Source: CAD feature listing. Evaluate the final solid. Frame: model axes, mm. A direction names the side the tool comes from. Round coordinates to 2 decimals unless told otherwise and drop trailing zeros. Loops run counter-clockwise (first coordinate to the right, second up) from the corner with the lowest first, then second, coordinate; pieces in that order, holes last. Notation, with made-up numbers: (-16, 49.5) - (6, 49.5) arc R20 cw to (6, 58.5) - close; hole circle Ø8 at (-30.5, 77.5). An arc over 180 degrees is marked (long way). One line per question, with ' | ' between items.
from build123d import *

# Parameters (mm, degrees)
SKIZZE1_W                       = 168
SKIZZE1_H                       = 60
AUFSATZ_LINEAR_AUSTRAGEN1_DEPTH = 10
SKIZZE2_R                       = 14
SCHNITT_LINEAR_AUSTRAGEN1_DEPTH = 27
SKIZZE3_R                       = 16
SCHNITT_LINEAR_AUSTRAGEN2_DEPTH = 8
SKIZZE4_R                       = 11
SCHNITT_LINEAR_AUSTRAGEN3_DEPTH = 21.6
SKIZZE5_W                       = 168
SKIZZE5_H                       = 10
AUFSATZ_LINEAR_AUSTRAGEN2_DEPTH = 50
SKIZZE6_R                       = 2
SCHNITT_LINEAR_AUSTRAGEN4_DEPTH = 10
SKIZZE7_R                       = 2.5
SCHNITT_LINEAR_AUSTRAGEN5_DEPTH = 10
SKIZZE8_R                       = 1.5
SCHNITT_LINEAR_AUSTRAGEN6_DEPTH = 27
FASE1_SIZE                      = 2
FASE2_SIZE                      = 2
FASE3_SIZE                      = 2
FASE4_SIZE                      = 2


with BuildPart() as part:
    # Skizze1 → Aufsatz-Linear austragen1 (new body)
    with BuildSketch(Plane.XY):
        with Locations((84, 30)):
            Rectangle(SKIZZE1_W, SKIZZE1_H)
    extrude(amount=AUFSATZ_LINEAR_AUSTRAGEN1_DEPTH)

    # Skizze2 → Schnitt-Linear austragen1 (cut)
    with BuildSketch(Plane.XY.offset(10)):
        with Locations((108, 32.5)):
            Circle(SKIZZE2_R)
    extrude(amount=-SCHNITT_LINEAR_AUSTRAGEN1_DEPTH, mode=Mode.SUBTRACT)

    # Skizze3 → Schnitt-Linear austragen2 (cut)
    with BuildSketch(Plane.XY.offset(10)):
        with Locations((108, 32.5)):
            Circle(SKIZZE3_R)
    extrude(amount=-SCHNITT_LINEAR_AUSTRAGEN2_DEPTH, mode=Mode.SUBTRACT)

    # Skizze4 → Schnitt-Linear austragen3 (cut)
    with BuildSketch(Plane(origin=(0, 0, 0), x_dir=(-1, 0, 0), z_dir=(0, 0, -1))):
        with Locations((-66, 32.50089026)):
            Circle(SKIZZE4_R)
    extrude(amount=-SCHNITT_LINEAR_AUSTRAGEN3_DEPTH, mode=Mode.SUBTRACT)

    # Skizze5 → Aufsatz-Linear austragen2 (add)
    with BuildSketch(Plane(origin=(0, 0, 0), x_dir=(-1, 0, 0), z_dir=(0, 0, -1))):
        with Locations((-84, 5)):
            Rectangle(SKIZZE5_W, SKIZZE5_H)
    extrude(amount=AUFSATZ_LINEAR_AUSTRAGEN2_DEPTH)

    # Skizze6 → Schnitt-Linear austragen4 (cut)
    with BuildSketch(Plane(origin=(0, 10, 0), x_dir=(1, 0, 0), z_dir=(0, 1, 0))):
        with Locations((5.5, 13.5)):
            Circle(SKIZZE6_R)
        with Locations((31.5, 13.5)):
            Circle(SKIZZE6_R)
        with Locations((162.5, 13.5)):
            Circle(SKIZZE6_R)
        with Locations((136.5, 13.5)):
            Circle(SKIZZE6_R)
    extrude(amount=-SCHNITT_LINEAR_AUSTRAGEN4_DEPTH, mode=Mode.SUBTRACT)

    # Skizze7 → Schnitt-Linear austragen5 (cut)
    with BuildSketch(Plane(origin=(0, 10, 0), x_dir=(1, 0, 0), z_dir=(0, 1, 0))):
        with Locations((104, 20)):
            Circle(SKIZZE7_R)
        with Locations((64, 20)):
            Circle(SKIZZE7_R)
        with Locations((64, 5)):
            Circle(SKIZZE7_R)
        with Locations((104, 5)):
            Circle(SKIZZE7_R)
    extrude(amount=-SCHNITT_LINEAR_AUSTRAGEN5_DEPTH, mode=Mode.SUBTRACT)

    # Skizze8 → Schnitt-Linear austragen6 (cut)
    with BuildSketch(Plane(origin=(0, 0, 0), x_dir=(-1, 0, 0), z_dir=(0, 0, -1))):
        with Locations((-50.5, 48)):
            Circle(SKIZZE8_R)
        with Locations((-50.5, 17)):
            Circle(SKIZZE8_R)
        with Locations((-81.5, 17)):
            Circle(SKIZZE8_R)
        with Locations((-81.5, 48)):
            Circle(SKIZZE8_R)
    extrude(amount=-SCHNITT_LINEAR_AUSTRAGEN6_DEPTH, mode=Mode.SUBTRACT)

    # Fase1
    fase1_edges = [part.edges().sort_by_distance(p)[0] for p in [
        (61.5, 10, -5),
    ]]
    chamfer(fase1_edges, length=FASE1_SIZE)

    # Fase2
    fase2_edges = [part.edges().sort_by_distance(p)[0] for p in [
        (61.5, 10, -20),
    ]]
    chamfer(fase2_edges, length=FASE2_SIZE)

    # Fase3
    fase3_edges = [part.edges().sort_by_distance(p)[0] for p in [
        (101.5, 10, -20),
    ]]
    chamfer(fase3_edges, length=FASE3_SIZE)

    # Fase4
    fase4_edges = [part.edges().sort_by_distance(p)[0] for p in [
        (101.5, 10, -5),
    ]]
    chamfer(fase4_edges, length=FASE4_SIZE)


solid = part.part
1. Section query B-B, the plane x = 162.5. Return loops of the section in (y, z), plus the area to 3 significant figures.
Worked out:
outline: (0, -50) - (10, -50) - (10, -15.5) - (0, -15.5) - close; (0, -11.5) - (10, -11.5) - (10, 0) - (60, 0) - (60, 10) - (0, 10) - close | area: 1,060 mm2
2. Contact query for flat-ended pins moving along their axis: P1, Ø4.5, axis at x = 64, z = -5, coming from the -Y side; P2, Ø16, axis at x = 104.5, y = 25.5, coming from the +Z side; P3, Ø4.5, axis at x = 5.5, z = -13.5, coming from the +Y side; P4, Ø25, axis at x = 66, y = 23, coming from the -Z side. Output: stop coordinate, or through.
Worked out:
P1: passes through | P2: stops at z = 2 | P3: stops at y = 10 | P4: stops at z = 0
3. Mould query, pull axis X, two halves, no side actions, for faces 3 (the flat face through (0, 16.2, 0.4)), 4 (the flat face through (83, 30, 10)), 5 (the cylindrical face through (80, 17, 5)). Classes: released by +X, released by -X, zero draft, split by the parting line, or undercut.
Worked out:
face 3: released by -X | face 4: zero draft | face 5: undercut
4. Section query C-C, the plane z = -30.5. Return loops of the section in (x, y), plus the area to 3 significant figures.
Worked out:
outline: (0, 0) - (168, 0) - (168, 10) - (0, 10) - close | area: 1,680 mm2
5. Access query for faces 1 (the flat face through (108, 18, 2)), 2 (the cylindrical face through (33.408, 5.07, -14.101)). Directions: +Z, -Z, +X, -X, +Y, -Y. A direction counts if a zero-diameter tool reaches every point of the face in a straight line with its end or side. Return the directions, or none.
Worked out:
face 1: +Z | face 2: +Y, -Y
6. Section query A-A, the plane z = -5. Return loops of the section in (x, y), plus the area to 3 significant figures.
Worked out:
outline: (0, 0) - (61.5, 0) - (61.5, 8) - (59.5, 10) - (0, 10) - close; (66.5, 0) - (101.5, 0) - (101.5, 8) - (99.5, 10) - (68.5, 10) - (66.5, 8) - close; (106.5, 0) - (168, 0) - (168, 10) - (108.5, 10) - (106.5, 8) - close | area: 1,570 mm2
7. Material intervals for probe 1 along Z at (x, y) = (104, 5.5); probe 2 along X at (y, z) = (6, -13.5); probe 3 along X at (y, z) = (2.5, -20), sorted ascending.
Worked out:
probe 1: z = -50 to -22.5, -17.5 to -7.5, -2.5 to 10 | probe 2: x = 0 to 3.5, 7.5 to 29.5, 33.5 to 134.5, 138.5 to 160.5, 164.5 to 168 | probe 3: x = 0 to 61.5, 66.5 to 101.5, 106.5 to 168
